Part model, mm, in its own coordinate system. Face numbers are marked on the shaded views. A direction names the side the tool comes from. Give positions to 0.01 mm unless a question says otherwise; leave off trailing zeros. Write each loop counter-clockwise with the first axis right and the second up, starting at its lowest first coordinate (ties: lowest second). Pieces come first, ordered by that corner, then holes. Notation, with made-up numbers: M -28,84 L 22,84 A33 ccw 22,120 Z; hole C -3,82 d7. An arc over 180 degrees is marked long. Use CSV: the item, a comma, the result in double quotes. Start each with the question number.
Item 1: Cut at D-D (y = 2.75). List the corners of the cut face in (x, z), then the cut area to 3 significant figures.
Item 2: Cut at C-C (y = 23.75). List the corners of the cut face in (x, z), then the cut area to 3 significant figures.
Item 3: Pin check, flat tips, straight feed: pin 1 (4 mm diameter, centred on x = -20, y = 24, fed in from -Z); pin 2 (2 mm diameter, centred on y = 15.5, z = 13, fed in from -X); pin 3 (8 mm diameter, centred on x = -16, y = 15, fed in from +Z); pin 4 (2 mm diameter, centred on x = -4, z = 28, fed in from -Y). Stop position of each tip, or through.
Item 4: Which spindle directions (+Z, -Z, +X, -X, +Y, -Y) get a long thin tool onto all of the face, cutting with end or side? Do the marked faces 1, 2 and 3. Say none if no direction does.
Item 5: Drill centre lines: line 1 (Y direction, x = -18, z = 2.5); line 2 (Z direction, x = -15.5, y = 6); line 3 (Z direction, x = 5.5, y = 25.75). Where is each one in solid material? Low to high. Write a range as [from, to].
Item 6: Cut at B-B (z = 14.5). List the corners of the cut face in (x, y).
Item 7: Cut at A-A (x = -19). List the corners of the cut face in (y, z).
from build123d import *

# Parameters (mm, degrees)
EXTRUDE_1_DEPTH     = 30
CUT_EXTRUDE_1_DEPTH = 24
SKETCH_3_W          = 29.306250819
SKETCH_3_H          = 11.935792743
CUT_EXTRUDE_2_DEPTH = 10


with BuildPart() as part:
    # 草图1 → 凸台-拉伸1 (new body)
    with BuildSketch(Plane(origin=(0, 0, 0), x_dir=(1, 0, 0), z_dir=(0, 1, 0))):
        Polygon((-37.717889908, 18.188073394), (-37.717889908, -25.940366972), (8.348623853, -25.940366972), (8.348623853, -36.972477064), (27.282110092, -36.972477064), (27.282110092, 28.027522936), (4.548530182, 28.027522936), (4.548530182, 18.188073394), align=None)
    extrude(amount=EXTRUDE_1_DEPTH)

    # 草图2 → 切除-拉伸1 (cut)
    with BuildSketch(Plane.XY.offset(25.940366972)):
        Polygon((-37.717889908, 25.912398035), (-8.411639089, 25.912398035), (-8.411639089, 11.935792743), (-20.845998279, 11.935792743), (-37.717889908, 0), align=None)
    extrude(amount=-CUT_EXTRUDE_1_DEPTH, mode=Mode.SUBTRACT)

    # 草图3 → 切除-拉伸2 (cut)
    with BuildSketch(Plane.XY.offset(25.940366972)):
        with Locations((-23.064764499, 5.967896372)):
            Rectangle(SKETCH_3_W, SKETCH_3_H)
    extrude(amount=-CUT_EXTRUDE_2_DEPTH, mode=Mode.SUBTRACT)


solid = part.part
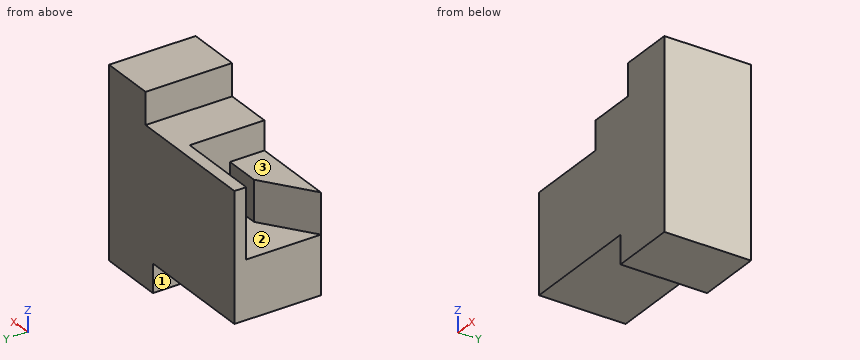
Worked answers:
1,outline,"M -37.72,-18.19 L 4.55,-18.19 L 4.55,-28.03 L 27.28,-28.03 L 27.28,36.97 L 8.35,36.97 L 8.35,25.94 L -8.41,25.94 L -8.41,15.94 L -33.83,15.94 L -33.83,1.94 L -37.72,1.94 Z"
1,area,"2,950 mm^2"
2,outline,"M -37.72,-18.19 L 4.55,-18.19 L 4.55,-28.03 L 27.28,-28.03 L 27.28,36.97 L 8.35,36.97 L 8.35,25.94 L -8.41,25.94 L -8.41,1.94 L -37.72,1.94 Z"
2,area,"2,600 mm^2"
3,pin 1,"stops at z = -18.19"
3,pin 2,"stops at x = -8.41"
3,pin 3,"stops at z = 15.94"
3,pin 4,"passes through"
4,face 1,"-Z, -X, +Y, -Y"
4,face 2,"+Z, -X"
4,face 3,"+Z, -X, -Y"
5,line 1,"y = [0, 11.94], [25.91, 30]"
5,line 2,"z = [-18.19, 15.94]"
5,line 3,"z = [-28.03, 25.94]"
6,outline,"M -37.72,0 L 27.28,0 L 27.28,30 L -37.72,30 L -37.72,25.91 L -8.41,25.91 L -8.41,11.94 L -20.85,11.94 Z"
7,outline,"M 0,-18.19 L 30,-18.19 L 30,25.94 L 25.91,25.94 L 25.91,1.94 L 11.94,1.94 L 11.94,15.94 L 0,15.94 Z"
